```python
from build123d import *

# Parameters (mm, degrees)
SKETCH1_R               = 150
BOSS_EXTRUDE1_DEPTH     = 5
CUT_EXTRUDE1_DEPTH      = 213.190951739
CUT_EXTRUDE1_DEPTH_BACK = 213.190951739
SKETCH2_R               = 6
CUT_EXTRUDE2_DEPTH      = 213.190951739
CUT_EXTRUDE2_DEPTH_BACK = 213.190951739
SKETCH3_R               = 3
CUT_EXTRUDE3_DEPTH      = 213.190951739
CUT_EXTRUDE3_DEPTH_BACK = 213.190951739
SKETCH5_R               = 3
SKETCH5_R_2             = 2
BOSS_EXTRUDE2_DEPTH     = 9.8
CIRPATTERN1_COUNT       = 4


with BuildPart() as part:
    # Sketch1 → Boss-Extrude1 (new body)
    with BuildSketch(Plane(origin=(0, 0, 0), x_dir=(1, 0, 0), z_dir=(0, 1, 0))):
        with Locations(Location((0, 0, 0), (0, 0, 270))):
            Circle(SKETCH1_R)
    extrude(amount=BOSS_EXTRUDE1_DEPTH)

    # Sketch2 → Cut-Extrude1 (cut, two sides: drawn at the far end of the back side and taken through both)
    with BuildSketch(Plane(origin=(0, 5, 0), x_dir=(1, 0, 0), z_dir=(0, 1, 0)).offset(-CUT_EXTRUDE1_DEPTH_BACK)):
        with Locations(Location((0, 0, 0), (0, 0, 270))):
            Circle(SKETCH2_R)
    extrude(amount=CUT_EXTRUDE1_DEPTH + CUT_EXTRUDE1_DEPTH_BACK, mode=Mode.SUBTRACT)

    # Sketch3 → Cut-Extrude2 (cut, two sides: drawn at the far end of the back side and taken through both)
    with BuildSketch(Plane(origin=(0, 5, 0), x_dir=(1, 0, 0), z_dir=(0, 1, 0)).offset(-CUT_EXTRUDE2_DEPTH_BACK)):
        with Locations(Location((-64.951905284, 37.5, 0), (0, 0, 270))):
            Circle(SKETCH3_R)
        with Locations(Location((64.951905284, 37.5, 0), (0, 0, 270))):
            Circle(SKETCH3_R)
        with Locations(Location((0, -75, 0), (0, 0, 270))):
            Circle(SKETCH3_R)
    extrude(amount=CUT_EXTRUDE2_DEPTH + CUT_EXTRUDE2_DEPTH_BACK, mode=Mode.SUBTRACT)

    # Sketch4 → Cut-Extrude3 (cut, two sides: drawn at the far end of the back side and taken through both)
    with BuildSketch(Plane(origin=(0, 5, 0), x_dir=(1, 0, 0), z_dir=(0, 1, 0)).offset(-CUT_EXTRUDE3_DEPTH_BACK)):
        with BuildLine():
            ThreePointArc((20.5, 148.592563744), (0, 150), (-20.5, 148.592563744))
            Line((-20.5, 148.592563744), (-20.5, 128.592563744))
            Line((-20.5, 128.592563744), (20.5, 128.592563744))
            Line((20.5, 128.592563744), (20.5, 148.592563744))
        make_face()
        with BuildLine():
            ThreePointArc((-148.592563744, 20.5), (-150, 0), (-148.592563744, -20.5))
            Line((-148.592563744, -20.5), (-128.592563744, -20.5))
            Line((-128.592563744, -20.5), (-128.592563744, 20.5))
            Line((-128.592563744, 20.5), (-148.592563744, 20.5))
        make_face()
        with BuildLine():
            Line((128.592563744, -20.5), (148.592563744, -20.5))
            ThreePointArc((148.592563744, -20.5), (149.647727282, -10.274128635), (150, 0))
            ThreePointArc((150, 0), (149.647727282, 10.274128635), (148.592563744, 20.5))
            Line((148.592563744, 20.5), (128.592563744, 20.5))
            Line((128.592563744, 20.5), (128.592563744, -20.5))
        make_face()
        with BuildLine():
            Line((-20.5, -128.592563744), (-20.5, -148.592563744))
            ThreePointArc((-20.5, -148.592563744), (0, -150), (20.5, -148.592563744))
            Line((20.5, -148.592563744), (20.5, -128.592563744))
            Line((20.5, -128.592563744), (-20.5, -128.592563744))
        make_face()
    extrude(amount=CUT_EXTRUDE3_DEPTH + CUT_EXTRUDE3_DEPTH_BACK, mode=Mode.SUBTRACT)

    # Sketch5 → Boss-Extrude2 (add, symmetric)
    # profile 1 of 2: a face of its own
    with BuildSketch(Plane.XY):
        with BuildLine():
            Line((-125.592563744, 0), (-128.592563744, 0))
            ThreePointArc((-128.592563744, 0), (-126.4712434, -0.878679656), (-125.592563744, -3))
            Line((-125.592563744, -3), (-125.592563744, 0))
        make_face()
    # profile 2 of 2: a face of its own
    with BuildSketch(Plane.XY):
        with Locations((-128.592563744, -3)):
            Circle(SKETCH5_R)
        with Locations((-128.592563744, -3)):
            Circle(SKETCH5_R_2, mode=Mode.SUBTRACT)
    boss_extrude2 = extrude(amount=BOSS_EXTRUDE2_DEPTH, both=True)

    # CirPattern1: Boss-Extrude2 ×4 about axis
    cirpattern1_axis = Axis((0, 0, 0), (0, 1, 0))
    for i in range(1, CIRPATTERN1_COUNT):
        add(boss_extrude2.rotate(cirpattern1_axis, i * 360 / CIRPATTERN1_COUNT))


solid = part.part
```
Can you work these out from the model? Positions are in its coordinate system, mm. Give positions to 0.01 mm unless a question says otherwise; leave off trailing zeros. Loops run counter-clockwise (first coordinate to the right, second up) from the corner with the lowest first, then second, coordinate; pieces in that order, holes last. Notation, with made-up numbers: M -27,27 L -22,27 A16 ccw -22,38 Z; hole C 9.5,72 d10. An arc over 180 degrees is marked long. Use one line per item in the form item = value. Start each with the question number.
(1) I want a section at C-C, the plane z = 95.5. Write out the boundary of the cut face in (x, y), and give its area (3 significant figures).
(2) I want a section at A-A, the plane y = 2.75. Write out the boundary of the cut face in (x, z), and give its area (3 significant figures).
(3) Thinking about a two-plate mould opening in X: for faces 1 (the cylindrical face through (105.099, 2.465, 107.024)), 2 (the cylindrical face through (-105.099, 2.465, -107.024)), 3 (the cylindrical face through (1.802, 2.465, 5.723)), which applies, released by +X, released by -X, zero draft, split by the parting line, or undercut?
(4) I'm going to push flat-ended pins straight in: P1, Ø5.5, axis at x = 0.5, y = 3, coming from the -Z side; P2, Ø1.5, axis at y = 1.5, z = -6.5, coming from the -X side; P3, Ø3, axis at y = -3, z = -128.59, coming from the -X side; P4, Ø3.5, axis at x = 0, y = -2, coming from the +Z side. Where does each tip first touch, or does it pass through?
(5) Please list where these lines run through material, in increasing order: line 1 (Z direction, x = 0, y = 2.1); line 2 (X direction, y = 1.9, z = 0); line 3 (Y direction, x = 59.5, z = -77).
(6) I want a section at B-B, the plane x = 90.5. Write out the boundary of the cut face in (y, z).
Worked out:
q1.outline = M -115.67,0 L 115.67,0 L 115.67,5 L -115.67,5 Z
q1.area = 1,160 mm²
q2.outline = M -148.59,-20.5 A150 ccw -20.5,-148.59 L -20.5,-128.59 L 20.5,-128.59 L 20.5,-148.59 A150 ccw 148.59,-20.5 L 128.59,-20.5 L 128.59,20.5 L 148.59,20.5 A150 ccw 20.5,148.59 L 20.5,128.59 L -20.5,128.59 L -20.5,148.59 A150 ccw -148.59,20.5 L -128.59,20.5 L -128.59,-20.5 Z; hole C -64.95,-37.5 d6; hole C 0,0 d12; hole C 0,75 d6; hole C 64.95,-37.5 d6
q2.area = 67,100 mm²
q3.face_1 = released by +X
q3.face_2 = released by -X
q3.face_3 = undercut
q4.P1 = -128.59
q4.P2 = -128.59
q4.P3 = through
q4.P4 = 131.59
q5.line_1 = -128.59 to -6, 6 to 72, 78 to 128.59
q5.line_2 = -128.59 to -6, 6 to 128.59
q5.line_3 = 0 to 5
q6.outline = M 0,-119.62 L 5,-119.62 L 5,119.62 L 0,119.62 Z
